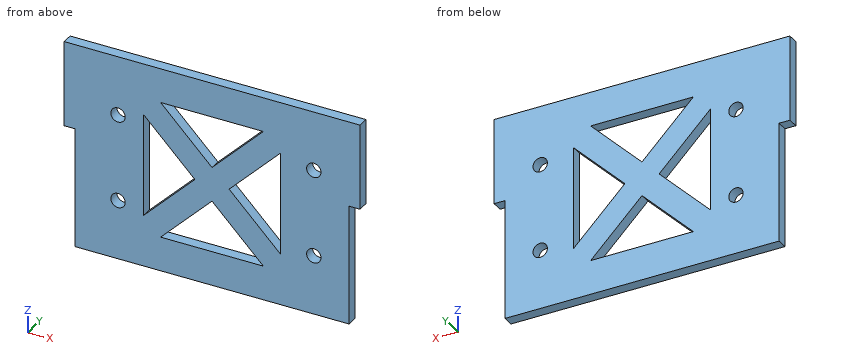
```python
from build123d import *

# Parameters (mm, degrees)
BOSS_EXTRUDE1_DEPTH = 3.175
SKETCH2_R           = 2.1
CUT_EXTRUDE1_DEPTH  = 3.175
CUT_EXTRUDE2_DEPTH  = 3.175


with BuildPart() as part:
    # Sketch1 → Boss-Extrude1 (new body)
    with BuildSketch(Plane(origin=(0, 0, 0), x_dir=(1, 0, 0), z_dir=(0, 1, 0))):
        Polygon((-43.175, -5), (-43.175, -30), (43.175, -30), (43.175, -5), (40, -5), (40, 30), (-40, 30), (-40, -5), align=None)
    extrude(amount=BOSS_EXTRUDE1_DEPTH)

    # Sketch2 → Cut-Extrude1 (cut)
    with BuildSketch(Plane(origin=(0, 3.175, 0), x_dir=(1, 0, 0), z_dir=(0, 1, 0))):
        with Locations(Location((-27.43, 12.7, 0), (0, 0, 270))):
            Circle(SKETCH2_R)
        with Locations(Location((29.72, 12.7, 0), (0, 0, 270))):
            Circle(SKETCH2_R)
        with Locations(Location((29.72, -12.7, 0), (0, 0, 270))):
            Circle(SKETCH2_R)
        with Locations(Location((-27.43, -12.7, 0), (0, 0, 270))):
            Circle(SKETCH2_R)
    extrude(amount=-CUT_EXTRUDE1_DEPTH, mode=Mode.SUBTRACT)

    # Sketch3 → Cut-Extrude2 (cut)
    with BuildSketch(Plane(origin=(0, 3.175, 0), x_dir=(1, 0, 0), z_dir=(0, 1, 0))):
        Polygon((-20, -15), (-20, 15), (-5, 0), align=None)
        Polygon((0, 5), (-15, 20), (15, 20), align=None)
        Polygon((5, 0), (20, 15), (20, -15), align=None)
        Polygon((0, -5), (15, -20), (-15, -20), align=None)
    extrude(amount=-CUT_EXTRUDE2_DEPTH, mode=Mode.SUBTRACT)


solid = part.part
```
The listing builds one solid part. Answer for the finished solid, in the listing's coordinates (mm). Round coordinates to 2 decimals unless told otherwise and drop trailing zeros. Loops run counter-clockwise (first coordinate to the right, second up) from the corner with the lowest first, then second, coordinate; pieces in that order, holes last.
Q1. Section A-A, the plane x = -27.43 is taken. Determine the outline of the cut face in (y, z) (3 decimals).
Q2. Find the intervals of material crossed by line 1 (X direction, y = 2.35, z = -12.7); line 2 (X direction, y = 1.3, z = 12.7) (3 decimals); line 3 (Z direction, x = -9, y = 1), in increasing order.
Q3. Section B-B, the plane z = 12.7 is taken. Determine the outline of the cut face in (x, y) (3 decimals), then the cut area to 3 significant figures.
Q4. Section C-C, the plane x = -7.5 is taken. Determine the outline of the cut face in (y, z) (3 decimals).
Q5. Section D-D, the plane y = 2.25 is taken. Count the separate pieces of the cut face and the enclosed holes in it, then the cut area to 3 significant figures.
Q6. Given pin 1 Ø1.6 at (x, y) = (41.5, 2.5) entering from -Z; pin 2 Ø1.5 at (y, z) = (0.5, 2.5) entering from +X; pin 3 Ø3.5 at (x, z) = (-27.43, 12.7) entering from -Y, each flat-ended and moving along its own axis, determine where each tip first touches the part or whether it passes through.
Completed:
1. outline: (0, -30) - (3.175, -30) - (3.175, -14.8) - (0, -14.8) - close; (0, -10.6) - (3.175, -10.6) - (3.175, 10.6) - (0, 10.6) - close; (0, 14.8) - (3.175, 14.8) - (3.175, 30) - (0, 30) - close
2. line 1: x = -40 to -29.53, -25.33 to -20, -17.7 to -7.7, 7.7 to 17.7, 20 to 27.62, 31.82 to 40
2. line 2: x = -43.175 to -29.53, -25.33 to -20, -17.7 to -7.7, 7.7 to 17.7, 20 to 27.62, 31.82 to 43.175
2. line 3: z = -30 to -20, -14 to -4, 4 to 14, 20 to 30
3. outline: (-43.175, 0) - (-29.53, 0) - (-29.53, 3.175) - (-43.175, 3.175) - close; (-25.33, 0) - (-20, 0) - (-20, 3.175) - (-25.33, 3.175) - close; (-17.7, 0) - (-7.7, 0) - (-7.7, 3.175) - (-17.7, 3.175) - close; (7.7, 0) - (17.7, 0) - (17.7, 3.175) - (7.7, 3.175) - close; (20, 0) - (27.62, 0) - (27.62, 3.175) - (20, 3.175) - close; (31.82, 0) - (43.175, 0) - (43.175, 3.175) - (31.82, 3.175) - close
3. area: 184 mm2
4. outline: (0, -30) - (3.175, -30) - (3.175, -20) - (0, -20) - close; (0, -12.5) - (3.175, -12.5) - (3.175, -2.5) - (0, -2.5) - close; (0, 2.5) - (3.175, 2.5) - (3.175, 12.5) - (0, 12.5) - close; (0, 20) - (3.175, 20) - (3.175, 30) - (0, 30) - close
5. separate pieces: 1
5. enclosed holes: 8
5. area: 4,000 mm2
6. pin 1: stops at z = 5
6. pin 2: stops at x = 40
6. pin 3: passes through
